Source: three-view drawing plus pictorial views. Frame: mm from the lowest corner of the part. Give positions to 0.01 mm unless a question says otherwise; leave off trailing zeros. Loops run counter-clockwise (first coordinate to the right, second up) from the corner with the lowest first, then second, coordinate; pieces in that order, holes last. Notation, with made-up numbers: (-32, -29.5) - (25, -29.5) arc R18 ccw to (25, 0.5) - close; hole circle Ø2 at (16.25, 38). An arc over 180 degrees is marked (long way). Put each result on its own line as item: value.
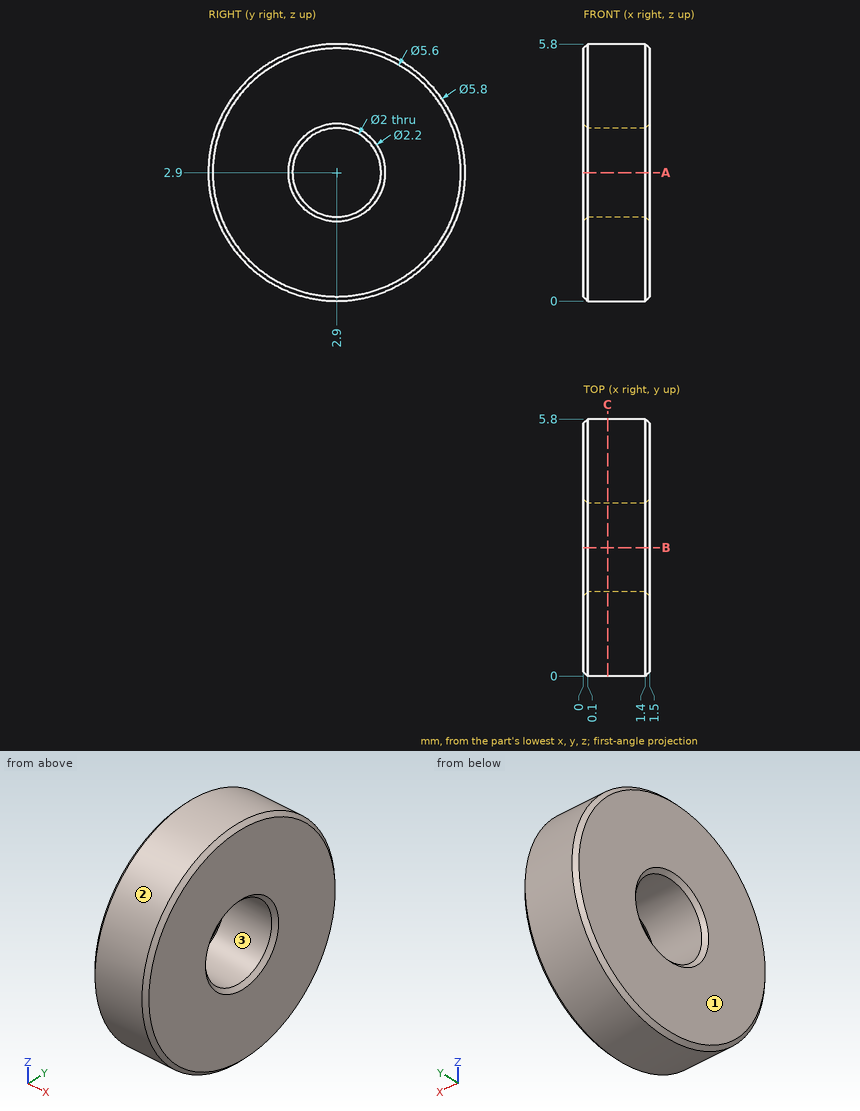
1) Section query A-A, the plane z = 2.9. Output: boundary loops of the cut face in (x, y), plus the area to 3 significant figures.
Check result:
outline: (0, 0.1) - (0.1, 0) - (1.4, 0) - (1.5, 0.1) - (1.5, 1.8) - (1.4, 1.9) - (0.1, 1.9) - (0, 1.8) - close; (0, 4) - (0.1, 3.9) - (1.4, 3.9) - (1.5, 4) - (1.5, 5.7) - (1.4, 5.8) - (0.1, 5.8) - (0, 5.7) - close
area: 5.66 mm²
2) Material intervals for line 1 along Y through (x, z) = (1.1, 2.9); line 2 along Z through (x, y) = (0.75, 2.35); line 3 along Y through (x, z) = (0.25, 3.5), sorted ascending. Write a range as [from, to].
Check result:
line 1: [0, 1.9], [3.9, 5.8]
line 2: [0.05, 2.06], [3.74, 5.75]
line 3: [0.06, 2.1], [3.7, 5.74]
3) Mould query, pull axis Y, two halves, no side actions, for the marked faces 1, 2 and 3. Classes: pulls with the +Y half, pulls with the -Y half, needs draft (parallel to the pull), parting line crosses it, or undercut.
Check result:
face 1: needs draft
face 2: parting line crosses it
face 3: undercut
4) Section query C-C, the plane x = 0.55. Output: boundary loops of the cut face in (y, z), plus the area to 3 significant figures.
Check result:
outline: circle Ø5.8 at (2.9, 2.9); hole circle Ø2 at (2.9, 2.9)
area: 23.3 mm²
